Here's how the part is built. I have some questions about the finished solid (model axes, mm). Give positions to 0.01 mm unless a question says otherwise; leave off trailing zeros. Write each loop counter-clockwise with the first axis right and the second up, starting at its lowest first coordinate (ties: lowest second). Pieces come first, ordered by that corner, then holes. Notation, with made-up numbers: (45.5, -27.75) -> (93.5, -27.75) arc R22 cw to (93.5, 8.25) -> close; hole circle Ø6 at (13, -2.5). An arc over 180 degrees is marked (long way). Use one line per item in the form item = value.
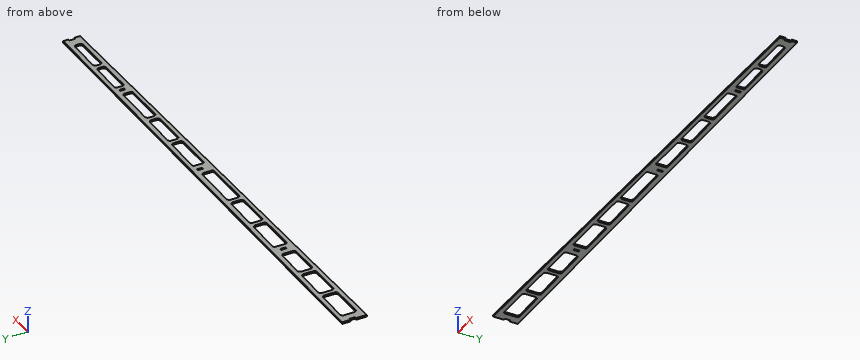
```python
from build123d import *

# Parameters (mm, degrees)
MODEL_W         = 2
MODEL_H         = 6
EXTRUDE_1_DEPTH = 2


with BuildPart() as part:
    # Model → 凸台-拉伸1 (new body)
    with BuildSketch(Plane.XY):
        Polygon((586.216263019, 41.768412003), (586.216263019, 35.855412003), (584.216263019, 35.855412003), (584.216263019, 29.154912003), (586.216263019, 29.154912003), (586.216263019, 22.750482518), (10.971476696, 13.842211299), (10.971476696, 25.978012003), (12.971476696, 25.978012003), (12.971476696, 32.006812003), (10.971476696, 32.006812003), (10.971476696, 41.768412003), (154.87521024, 41.768412003), (317.652575925, 41.768412003), (481.210656258, 41.768412003), align=None)
        with Locations((154.779030244, 29.144412003)):
            Rectangle(MODEL_W, MODEL_H, mode=Mode.SUBTRACT)
        Polygon((318.855190189, 33.150012003), (318.855190189, 30.095512003), (320.855190189, 30.095512003), (320.855190189, 36.095512003), (318.855190189, 36.095512003), align=None, mode=Mode.SUBTRACT)
        Polygon((480.71418574, 34.458512003), (480.71418574, 29.376512003), (482.71418574, 29.376512003), (482.71418574, 35.376512003), (480.71418574, 35.376512003), align=None, mode=Mode.SUBTRACT)
        with BuildLine():
            Line((58.757152566, 36.70165117), (24.257789514, 36.910650883))
            ThreePointArc((24.257789514, 36.910650883), (22.131185086, 36.044838231), (21.239670672, 33.928879822))
            Line((21.239670672, 33.928879822), (21.16943188, 22.334636165))
            ThreePointArc((21.16943188, 22.334636165), (22.051503861, 20.191700151), (24.197293169, 19.316592165))
            Line((24.197293169, 19.316592165), (58.699867458, 19.637667912))
            ThreePointArc((58.699867458, 19.637667912), (60.796713244, 20.519665053), (61.671896071, 22.619364132))
            Line((61.671896071, 22.619364132), (61.738923627, 33.683532329))
            ThreePointArc((61.738923627, 33.683532329), (60.873110975, 35.810136756), (58.757152566, 36.70165117))
        make_face(mode=Mode.SUBTRACT)
        with BuildLine():
            Line((146.748077677, 33.168540536), (146.688962862, 23.41052012))
            ThreePointArc((146.688962862, 23.41052012), (145.813780035, 21.310821041), (143.716934249, 20.4288239))
            Line((143.716934249, 20.4288239), (113.202550526, 20.144861652))
            ThreePointArc((113.202550526, 20.144861652), (111.056761218, 21.019969638), (110.174689236, 23.162905652))
            Line((110.174689236, 23.162905652), (110.236644098, 33.389729523))
            ThreePointArc((110.236644098, 33.389729523), (111.128158512, 35.505687932), (113.254762939, 36.371500584))
            Line((113.254762939, 36.371500584), (143.766306616, 36.186659378))
            ThreePointArc((143.766306616, 36.186659378), (145.882265025, 35.295144964), (146.748077677, 33.168540536))
        make_face(mode=Mode.SUBTRACT)
        with BuildLine():
            Line((69.756360643, 36.635017148), (102.25576428, 36.438133338))
            ThreePointArc((102.25576428, 36.438133338), (104.371722689, 35.546618924), (105.237535341, 33.420014496))
            Line((105.237535341, 33.420014496), (105.174556682, 23.024193324))
            ThreePointArc((105.174556682, 23.024193324), (104.299373855, 20.924494244), (102.202528069, 20.042497104))
            Line((102.202528069, 20.042497104), (69.700099353, 19.740034409))
            ThreePointArc((69.700099353, 19.740034409), (67.554310045, 20.615142396), (66.672238064, 22.75807841))
            Line((66.672238064, 22.75807841), (66.738241802, 33.653246087))
            ThreePointArc((66.738241802, 33.653246087), (67.629756216, 35.769204496), (69.756360643, 36.635017148))
        make_face(mode=Mode.SUBTRACT)
        with BuildLine():
            Line((163.541092581, 36.647103391), (202.093717488, 36.421153648))
            ThreePointArc((202.093717488, 36.421153648), (204.20886557, 35.527718408), (205.072747005, 33.400328739))
            Line((205.072747005, 33.400328739), (205.010197063, 24.421095996))
            ThreePointArc((205.010197063, 24.421095996), (204.134099679, 22.323185807), (202.038269411, 21.442124358))
            Line((202.038269411, 21.442124358), (163.465475762, 21.112553873))
            ThreePointArc((163.465475762, 21.112553873), (162.034270797, 21.69658021), (161.446857912, 23.12639856))
            Line((161.446857912, 23.12639856), (161.527209308, 34.661083712))
            ThreePointArc((161.527209308, 34.661083712), (162.122832802, 36.071182434), (163.541092581, 36.647103391))
        make_face(mode=Mode.SUBTRACT)
        with BuildLine():
            Line((213.082693343, 36.344603699), (248.994694933, 36.094438268))
            ThreePointArc((248.994694933, 36.094438268), (251.109843016, 35.201003028), (251.973724451, 33.073613359))
            Line((251.973724451, 33.073613359), (251.916500205, 24.858900378))
            ThreePointArc((251.916500205, 24.858900378), (251.040402821, 22.760990189), (248.944572553, 21.87992874))
            Line((248.944572553, 21.87992874), (213.036483972, 21.544777225))
            ThreePointArc((213.036483972, 21.544777225), (210.890640913, 22.419855058), (210.008539459, 24.56282045))
            Line((210.008539459, 24.56282045), (210.061850696, 33.362850376))
            ThreePointArc((210.061850696, 33.362850376), (210.954334175, 35.479765744), (213.082693343, 36.344603699))
        make_face(mode=Mode.SUBTRACT)
        with BuildLine():
            Line((259.984364938, 36.017883484), (309.946986323, 35.73855234))
            ThreePointArc((309.946986323, 35.73855234), (311.357085044, 35.142928847), (311.933006001, 33.724669067))
            Line((311.933006001, 33.724669067), (311.867917884, 24.38107371))
            ThreePointArc((311.867917884, 24.38107371), (311.289568546, 22.971847644), (309.886518402, 22.378672834))
            Line((309.886518402, 22.378672834), (259.93857923, 21.982545284))
            ThreePointArc((259.93857923, 21.982545284), (257.795454375, 22.859145292), (256.914842601, 25.000624832))
            Line((256.914842601, 25.000624832), (256.963522291, 33.03613016))
            ThreePointArc((256.963522291, 33.03613016), (257.85600577, 35.153045529), (259.984364938, 36.017883484))
        make_face(mode=Mode.SUBTRACT)
        with BuildLine():
            Line((329.559168481, 36.86823931), (370.143868366, 36.585523546))
            ThreePointArc((370.143868366, 36.585523546), (372.258059929, 35.693057805), (373.122915621, 33.567422443))
            Line((373.122915621, 33.567422443), (373.084136783, 27.166240277))
            ThreePointArc((373.084136783, 27.166240277), (372.209502307, 25.067091475), (370.113661797, 24.184558917))
            Line((370.113661797, 24.184558917), (329.500631729, 23.7855848))
            ThreePointArc((329.500631729, 23.7855848), (328.069426764, 24.369611137), (327.482013878, 25.799429487))
            Line((327.482013878, 25.799429487), (327.545285209, 34.882219631))
            ThreePointArc((327.545285209, 34.882219631), (328.140908702, 36.292318353), (329.559168481, 36.86823931))
        make_face(mode=Mode.SUBTRACT)
        with BuildLine():
            Line((381.143677955, 36.508898129), (417.045539961, 36.258803331))
            ThreePointArc((417.045539961, 36.258803331), (419.159731524, 35.36633759), (420.024587216, 33.240702227))
            Line((420.024587216, 33.240702227), (419.990439925, 27.604044659))
            ThreePointArc((419.990439925, 27.604044659), (419.115286475, 25.504375053), (417.018494535, 24.622349215))
            Line((417.018494535, 24.622349215), (381.113087215, 24.287222726))
            ThreePointArc((381.113087215, 24.287222726), (378.967244157, 25.162300559), (378.085142702, 27.305265951))
            Line((378.085142702, 27.305265951), (378.122835308, 33.527144806))
            ThreePointArc((378.122835308, 33.527144806), (379.015318787, 35.644060174), (381.143677955, 36.508898129))
        make_face(mode=Mode.SUBTRACT)
        with BuildLine():
            Line((428.04534955, 36.182177913), (472.3342856, 35.87365819))
            ThreePointArc((472.3342856, 35.87365819), (473.744384321, 35.278034697), (474.320305278, 33.859774917))
            Line((474.320305278, 33.859774917), (474.273385029, 27.12423169))
            ThreePointArc((474.273385029, 27.12423169), (473.689320106, 25.725624897), (472.292099928, 25.138250597))
            Line((472.292099928, 25.138250597), (428.019390357, 24.725027108))
            ThreePointArc((428.019390357, 24.725027108), (425.873547299, 25.600104941), (424.991445844, 27.743070333))
            Line((424.991445844, 27.743070333), (425.024506903, 33.20042459))
            ThreePointArc((425.024506903, 33.20042459), (425.916990382, 35.317339958), (428.04534955, 36.182177913))
        make_face(mode=Mode.SUBTRACT)
        with BuildLine():
            Line((489.48114747, 36.970903278), (524.086911809, 36.729837184))
            ThreePointArc((524.086911809, 36.729837184), (526.202059891, 35.836401944), (527.065941326, 33.709012275))
            Line((527.065941326, 33.709012275), (527.040585105, 30.069050249))
            ThreePointArc((527.040585105, 30.069050249), (526.164487721, 27.97114006), (524.068657453, 27.09007861))
            Line((524.068657453, 27.09007861), (489.48114747, 26.76725284))
            ThreePointArc((489.48114747, 26.76725284), (488.054336113, 27.346909518), (487.462481687, 28.768704459))
            Line((487.462481687, 28.768704459), (487.467264197, 34.9848836))
            ThreePointArc((487.467264197, 34.9848836), (488.062887691, 36.394982321), (489.48114747, 36.970903278))
        make_face(mode=Mode.SUBTRACT)
        with BuildLine():
            Line((535.08073548, 36.653253465), (570.987889254, 36.403121804))
            ThreePointArc((570.987889254, 36.403121804), (573.103037337, 35.509686564), (573.966918772, 33.382296895))
            Line((573.966918772, 33.382296895), (573.946888247, 30.506854631))
            ThreePointArc((573.946888247, 30.506854631), (573.070790863, 28.408944442), (570.974960595, 27.527882992))
            Line((570.974960595, 27.527882992), (535.066872014, 27.192731478))
            ThreePointArc((535.066872014, 27.192731478), (532.921028955, 28.067809311), (532.038927501, 30.210774703))
            Line((532.038927501, 30.210774703), (532.059892833, 33.671500141))
            ThreePointArc((532.059892833, 33.671500141), (532.952376312, 35.78841551), (535.08073548, 36.653253465))
        make_face(mode=Mode.SUBTRACT)
    extrude(amount=EXTRUDE_1_DEPTH)


solid = part.part
```
Q1. If I drill on line 1 along Y through (x, z) = (371.5, 1.3); line 2 along Y through (x, z) = (552.5, 1.75); line 3 along Y through (x, z) = (483, 0.75), over which ranges is the centre line in solid material (lowest first)? Write a range as from..to.
Result set:
line_1 = 19.43..24.54, 36.25..41.77
line_2 = 22.23..27.36, 36.53..41.77
line_3 = 21.15..41.77
Q2. Will these pins go through, and if not, where does the flat tip stop? pin 1 Ø1 at (y, z) = (33, 0.5) entering from +X; pin 2 Ø0.6 at (x, z) = (482, 1.5) entering from -Y; pin 3 Ø1 at (x, z) = (155, 1) entering from -Y.
Result set:
pin_1 = 584.22
pin_2 = 21.13
pin_3 = 16.06
Q3. I want a section at A-A, the plane x = 90. Write out the boundary of the cut face in (y, z), and give its area (3 significant figures).
Result set:
outline = (15.07, 0) -> (19.93, 0) -> (19.93, 2) -> (15.07, 2) -> close; (36.51, 0) -> (41.77, 0) -> (41.77, 2) -> (36.51, 2) -> close
area = 20.2 mm2
Q4. I want a section at B-B, the plane z = 0.4. Count the separate pieces of the cut face and the enclosed holes in it, and give its area (3 significant figures).
Result set:
separate_pieces = 1
enclosed_holes = 14
area = 7,160 mm2
Q5. I want a section at C-C, the plane x = 349. Write out the boundary of the cut face in (y, z).
Result set:
outline = (19.08, 0) -> (23.98, 0) -> (23.98, 2) -> (19.08, 2) -> close; (36.73, 0) -> (41.77, 0) -> (41.77, 2) -> (36.73, 2) -> close
